Study the drawing (mm; zero at the part's minimum x, y, z) and answer. Coordinates: 2 decimals unless noted, no trailing zeros. Order: outer loops, then holes, each group sorted by start corner. A loop starts at its lowest first (then second) coordinate and runs counter-clockwise, first axis right, second up. Notation, with made-up numbers: M -15.5,45.25 L 23.5,45.25 A18 ccw 23.5,50.25 Z; hole C 63.5,42 d4. An arc over 180 degrees is marked long. One line per item, written item: value. Start each with the question number.
Q1. Straight lines are drawn through the part: line 1 along X through (y, z) = (5, 15); line 2 along Y through (x, z) = (3.75, 13.5). For each, find the intervals that lie inside material, in ascending order. Write a range as [from, to].
Q2. The part is cut by section D-D on y = 1.25. Give the vertices of the cut face in (x, z), then the cut area to 3 significant figures.
Q3. The part is cut by section C-C on z = 34. Give the vertices of the cut face in (x, y), then the cut area to 3 significant figures.
Q4. The part is cut by section A-A on y = 5. Give the vertices of the cut face in (x, z), then the cut area to 3 significant figures.
Q5. Each of these flat-tipped pins is pushed along its axis until it touches: pin 1 Ø1 at (y, z) = (2.5, 21.5) entering from +X; pin 2 Ø2 at (x, y) = (5, 5) entering from -Z; pin 3 Ø1 at (y, z) = (3, 23) entering from +X. Where does it stop, or does it pass through?
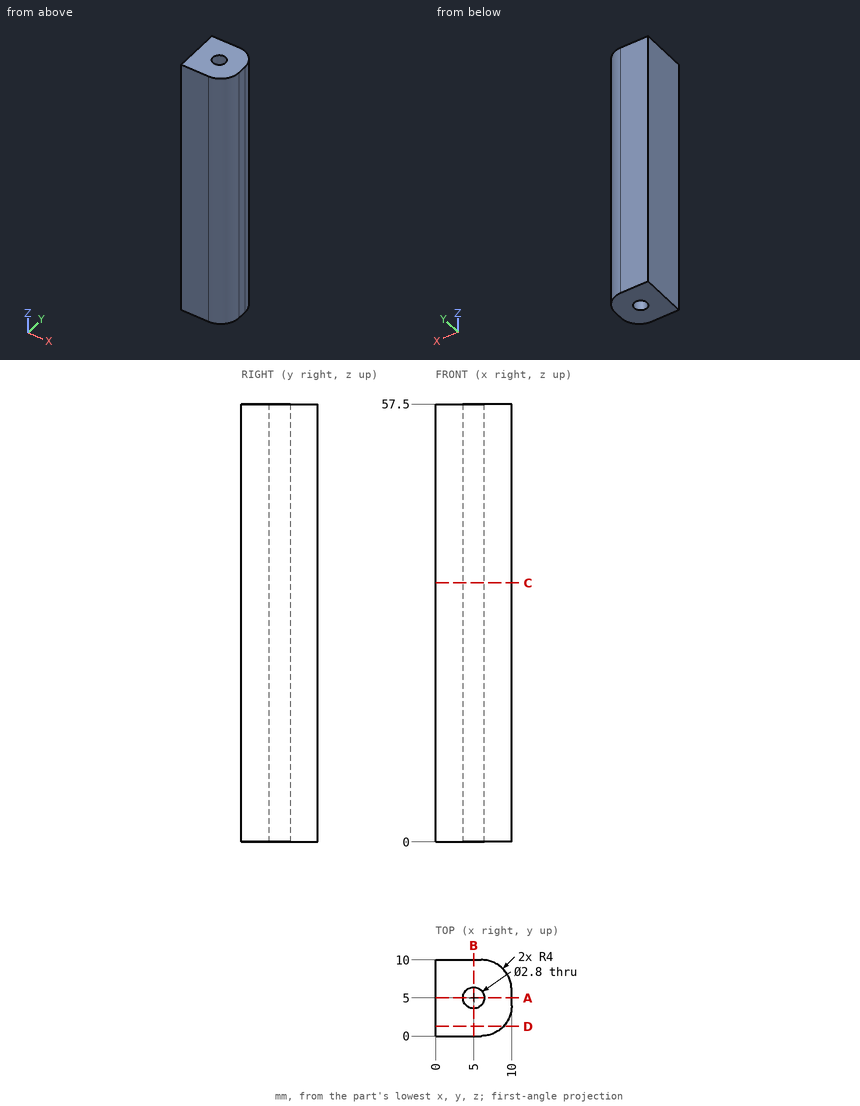
Output:
1. line 1: x = [0, 3.6], [6.4, 10]
1. line 2: y = [0, 4.37], [5.63, 10]
2. outline: M 0,0 L 8.9,0 L 8.9,57.5 L 0,57.5 Z
2. area: 512 mm^2
3. outline: M 0,0 L 6,0 A4 ccw 10,4 L 10,6 A4 ccw 6,10 L 0,10 Z; hole C 5,5 d2.8
3. area: 87.0 mm^2
4. outline: M 0,0 L 3.6,0 L 3.6,57.5 L 0,57.5 Z; M 6.4,0 L 10,0 L 10,57.5 L 6.4,57.5 Z
4. area: 414 mm^2
5. pin 1: stops at x = 9.87
5. pin 2: passes through
5. pin 3: stops at x = 9.97
